The listing builds one solid part. Answer for the finished solid, in the listing's coordinates (mm). A direction names the side the tool comes from. Give positions to 0.01 mm unless a question says otherwise; leave off trailing zeros. Order: outer loops, then holes, each group sorted by start corner. A loop starts at its lowest first (then second) coordinate and runs counter-clockwise, first axis right, second up. Notation, with made-up numbers: (87, -19) - (138, -19) arc R10 ccw to (138, -11) - close; hole circle Ø7 at (36.25, -34). An arc over 180 degrees is marked (long way). Answer in a Markdown table with one row per item.
from build123d import *


with BuildPart() as part:
    # Schizzo1 → Rivoluzione1 (revolve)
    with BuildSketch(Plane(origin=(0, 0, 0), x_dir=(0, 0, -1), z_dir=(1, 0, 0)), mode=Mode.PRIVATE) as rivoluzione1_sk:
        with BuildLine():
            Line((-73, 0), (-72, 0))
            Line((-72, 0), (-72, 3))
            Line((-72, 3), (-67, 3))
            Line((-67, 3), (-67, 17))
            Line((-67, 17), (-17.154700538, 17))
            Line((-17.154700538, 17), (-16, 19))
            Line((-16, 19), (-68, 19))
            ThreePointArc((-68, 19), (-68.707106781, 18.707106781), (-69, 18))
            Line((-69, 18), (-69, 6))
            Line((-69, 6), (-70, 5))
            Line((-70, 5), (-73, 5))
            Line((-73, 5), (-73, 0))
        make_face()
    revolve(rivoluzione1_sk.sketch.rotate(Axis((0, 0, 0), (0, 1, 0)), 180), axis=Axis((0, 0, 0), (0, 1, 0)))


solid = part.part
Item 1: Each of these flat-tipped pins is pushed along its axis until it touches: P1, Ø4, axis at x = 29, y = 14, coming from the -Z side; P2, Ø10, axis at x = 36.5, y = 13.5, coming from the +Z side; P3, Ø3, axis at x = 50.5, y = 5, coming from the -Z side. Where does it stop, or does it pass through?
Answer block:
| item | result |
|---|---|
| P1 | z = -63.5 |
| P2 | z = 61.39 |
| P3 | z = -54.11 |
Item 2: Find section B-B on z = 0. Write down the section's boundary in (x, y).
Answer block:
| item | result |
|---|---|
| outline | (-73, 0) - (-72, 0) - (-72, 3) - (-67, 3) - (-67, 17) - (-17.15, 17) - (-16, 19) - (-68, 19) arc R1 ccw to (-69, 18) - (-69, 6) - (-70, 5) - (-73, 5) - close; (16, 19) - (17.15, 17) - (67, 17) - (67, 3) - (72, 3) - (72, 0) - (73, 0) - (73, 5) - (70, 5) - (69, 6) - (69, 18) arc R1 ccw to (68, 19) - close |
Item 3: Which of the six approach directions +Z, -Z, +X, -X, +Y, -Y give full straight-line access (tool end or side, diameter ignored) to faces 5 (the face through (59, 5, 38)), 6 (the face through (14, 19, 14)), 7 (the face through (-48.66, 1.52, 53.07))?
Answer block:
| item | result |
|---|---|
| face 5 | +Y |
| face 6 | +Z, -Z, +X, -X, +Y |
| face 7 | -Y |
Item 4: Consider line 1 (X direction, y = 8.5, z = 0); line 2 (X direction, y = 1.4, z = 0); line 3 (Z direction, x = -1.5, y = 6). Determine where each line is inside the solid, lowest interval first.
Answer block:
| item | result |
|---|---|
| line 1 | -69 to -67, 67 to 69 |
| line 2 | -73 to -72, 72 to 73 |
| line 3 | -68.98 to -66.98, 66.98 to 68.98 |
Item 5: Determine the mould class of faces 1 (the face through (14, 17, -14)), 2 (the face through (64.76, 2.46, -33.69)), 3 (the face through (25.66, 10.1, -61.89)), 4 (the face through (48, 0, -54)) for opening direction X: pulls with the +X half, pulls with the -X half, needs draft (parallel to the pull), parting line crosses it, or undercut.
Answer block:
| item | result |
|---|---|
| face 1 | undercut |
| face 2 | parting line crosses it |
| face 3 | undercut |
| face 4 | needs draft |
Item 6: Find section C-C on y = 8.5. Write down the section's boundary in (x, z), then the cut area to 3 significant figures.
Answer block:
| item | result |
|---|---|
| outline | circle Ø138 at (0, 0); hole circle Ø134 at (0, 0) |
| area | 855 mm² |
Item 7: Find section A-A on x = 0. Write down the section's boundary in (y, z).
Answer block:
| item | result |
|---|---|
| outline | (0, -73) - (5, -73) - (5, -70) - (6, -69) - (18, -69) arc R1 ccw to (19, -68) - (19, -16) - (17, -17.15) - (17, -67) - (3, -67) - (3, -72) - (0, -72) - close; (0, 72) - (3, 72) - (3, 67) - (17, 67) - (17, 17.15) - (19, 16) - (19, 68) arc R1 ccw to (18, 69) - (6, 69) - (5, 70) - (5, 73) - (0, 73) - close |
